```python
from build123d import *
from build123d.topology import SkipClean

# Parameters (mm, degrees)
SKETCH_1_R      = 1.75
EXTRUDE_1_DEPTH = 3
EXTRUDE_START   = 4
SKETCH_2_R      = 9.1
SKETCH_2_R_2    = 7.1
EXTRUDE_2_DEPTH = 4
SKETCH_3_R      = 7.1
SKETCH_3_R_2    = 6.1
EXTRUDE_3_DEPTH = 2


with BuildPart() as part:
    # Эскиз1 → Бобышка-Вытянуть1 (new body)
    # profile 1 of 8: a face of its own
    with BuildSketch(Plane.XY):
        with BuildLine():
            Line((-16, 5), (-16, -5))
            Line((-16, -5), (-7.603288762, -5))
            ThreePointArc((-7.603288762, -5), (-9.1, 0), (-7.603288762, 5))
            Line((-7.603288762, 5), (-16, 5))
        make_face()
        with Locations((-12.5, 0)):
            Circle(SKETCH_1_R, mode=Mode.SUBTRACT)
    # profile 2 of 8: a face of its own
    with BuildSketch(Plane.XY):
        with BuildLine():
            ThreePointArc((-7.603288762, 5), (-9.1, 0), (-7.603288762, -5))
            Line((-7.603288762, -5), (-5.040833264, -5))
            ThreePointArc((-5.040833264, -5), (-7.1, 0), (-5.040833264, 5))
            Line((-5.040833264, 5), (-7.603288762, 5))
        make_face()
    # profile 3 of 8: a face of its own
    with BuildSketch(Plane.XY):
        with BuildLine():
            Line((5.040833264, -5), (7.603288762, -5))
            ThreePointArc((7.603288762, -5), (8.717795815, -2.609604593), (9.1, 0))
            ThreePointArc((9.1, 0), (8.717795815, 2.609604593), (7.603288762, 5))
            Line((7.603288762, 5), (5.040833264, 5))
            ThreePointArc((5.040833264, 5), (6.565055833, 2.703708918), (7.1, 0))
            ThreePointArc((7.1, 0), (6.565055833, -2.703708918), (5.040833264, -5))
        make_face()
    # profile 4 of 8: a face of its own
    with BuildSketch(Plane.XY):
        with BuildLine():
            ThreePointArc((7.603288762, 5), (0, 9.1), (-7.603288762, 5))
            Line((-7.603288762, 5), (-5.040833264, 5))
            ThreePointArc((-5.040833264, 5), (0, 7.1), (5.040833264, 5))
            Line((5.040833264, 5), (7.603288762, 5))
        make_face()
    # profile 5 of 8: a face of its own
    with BuildSketch(Plane.XY):
        with BuildLine():
            ThreePointArc((-7.603288762, 5), (-9.1, 0), (-7.603288762, -5))
            Line((-7.603288762, -5), (-5.040833264, -5))
            ThreePointArc((-5.040833264, -5), (-7.1, 0), (-5.040833264, 5))
            Line((-5.040833264, 5), (-7.603288762, 5))
        make_face()
    # profile 6 of 8: a face of its own
    with BuildSketch(Plane.XY):
        with BuildLine():
            Line((5.040833264, -5), (7.603288762, -5))
            ThreePointArc((7.603288762, -5), (8.717795815, -2.609604593), (9.1, 0))
            ThreePointArc((9.1, 0), (8.717795815, 2.609604593), (7.603288762, 5))
            Line((7.603288762, 5), (5.040833264, 5))
            ThreePointArc((5.040833264, 5), (6.565055833, 2.703708918), (7.1, 0))
            ThreePointArc((7.1, 0), (6.565055833, -2.703708918), (5.040833264, -5))
        make_face()
    # profile 7 of 8: a face of its own
    with BuildSketch(Plane.XY):
        with BuildLine():
            ThreePointArc((9.1, 0), (8.717795815, -2.609604593), (7.603288762, -5))
            Line((7.603288762, -5), (16, -5))
            Line((16, -5), (16, 5))
            Line((16, 5), (7.603288762, 5))
            ThreePointArc((7.603288762, 5), (8.717795815, 2.609604593), (9.1, 0))
        make_face()
        with Locations((12.5, 0)):
            Circle(SKETCH_1_R, mode=Mode.SUBTRACT)
    # profile 8 of 8: a face of its own
    with BuildSketch(Plane.XY):
        with BuildLine():
            Line((-5.040833264, -5), (-7.603288762, -5))
            ThreePointArc((-7.603288762, -5), (0, -9.1), (7.603288762, -5))
            Line((7.603288762, -5), (5.040833264, -5))
            ThreePointArc((5.040833264, -5), (0, -7.1), (-5.040833264, -5))
        make_face()
    extrude(amount=EXTRUDE_1_DEPTH)

    # Эскиз2 → Бобышка-Вытянуть2 (add)
    with SkipClean():  # the faces are left unmerged after this step: merging them gives an invalid solid
        with BuildSketch(Plane(origin=(0, 0, 0), x_dir=(-1, 0, 0), z_dir=(0, 0, -1)).offset(EXTRUDE_START)):
            Circle(SKETCH_2_R)
            Circle(SKETCH_2_R_2, mode=Mode.SUBTRACT)
        extrude(amount=-EXTRUDE_2_DEPTH)

    # Эскиз3 → Бобышка-Вытянуть3 (add)
    with SkipClean():  # the faces are left unmerged after this step: merging them gives an invalid solid
        with BuildSketch(Plane.XY.offset(-4)):
            Circle(SKETCH_3_R)
            Circle(SKETCH_3_R_2, mode=Mode.SUBTRACT)
        extrude(amount=EXTRUDE_3_DEPTH)


solid = part.part
```
Check sheet for the modelled part. Datum: model origin and axes. Units: mm. A direction names the side the tool comes from. Round coordinates to 2 decimals unless told otherwise and drop trailing zeros. Write each loop counter-clockwise with the first axis right and the second up, starting at its lowest first coordinate (ties: lowest second). Pieces come first, ordered by that corner, then holes. Notation, with made-up numbers: (40, -13.75) -> (93, -13.75) arc R23 cw to (93, 12.25) -> close; hole circle Ø4 at (14.5, 2). An arc over 180 degrees is marked (long way). Put each result on its own line as item: value.
(1) Sectioned sample at A-A (x = 12.5). Enter the section's corners in (y, z), plus the area to 3 significant figures.
Values found:
outline: (-5, 0) -> (-1.75, 0) -> (-1.75, 3) -> (-5, 3) -> close; (1.75, 0) -> (5, 0) -> (5, 3) -> (1.75, 3) -> close
area: 19.5 mm^2
(2) Sectioned sample at B-B (y = 3.25). Enter the section's corners in (x, z), plus the area to 3 significant figures.
Values found:
outline: (-16, 0) -> (-8.5, 0) -> (-8.5, -4) -> (-5.16, -4) -> (-5.16, -2) -> (-6.31, -2) -> (-6.31, 3) -> (-16, 3) -> close; (5.16, -4) -> (8.5, -4) -> (8.5, 0) -> (16, 0) -> (16, 3) -> (6.31, 3) -> (6.31, -2) -> (5.16, -2) -> close
area: 80.2 mm^2
(3) Go/stop test with flat-tipped pins: pin 1 Ø4 at (x, y) = (-12.5, 0) entering from -Z; pin 2 Ø0.9 at (x, z) = (-13, 1.5) entering from +Y; pin 3 Ø3 at (x, y) = (12.5, 0) entering from -Z; pin 4 Ø4 at (y, z) = (7, -2) entering from -X. Record where each tip stops, or that it passes through.
Values found:
pin 1: stops at z = 0
pin 2: stops at y = 5
pin 3: passes through
pin 4: stops at x = -7.6
(4) Material ranges on line 1 (Y direction, x = 12.5, z = 1.55); line 2 (X direction, y = 1, z = 1); line 3 (X direction, y = 6, z = 2.5), recorded low to high.
Values found:
line 1: y = -5 to -1.75, 1.75 to 5
line 2: x = -16 to -13.94, -11.06 to -7.03, 7.03 to 11.06, 13.94 to 16
line 3: x = -6.84 to -3.8, 3.8 to 6.84
(5) Tool access check on faces 1 (the face through (-16, 0, 1)), 2 (the face through (12, -5, 1)), 3 (the face through (12, 5, 1)), 4 (the face through (16, 0, 1)), 5 (the face through (2, 6, -2)). Record the directions out of +Z, -Z, +X, -X, +Y, -Y that give a thin tool (end or side, any length) a straight path to the whole face; none if there is none.
Values found:
face 1: +Z, -Z, -X, +Y, -Y
face 2: +Z, -Z, +X, -Y
face 3: +Z, -Z, +X, +Y
face 4: +Z, -Z, +X, +Y, -Y
face 5: +Z
(6) Sectioned sample at D-D (y = 1). Enter the section's corners in (x, z).
Values found:
outline: (-16, 0) -> (-13.94, 0) -> (-13.94, 3) -> (-16, 3) -> close; (-11.06, 0) -> (-9.04, 0) -> (-9.04, -4) -> (-6.02, -4) -> (-6.02, -2) -> (-7.03, -2) -> (-7.03, 3) -> (-11.06, 3) -> close; (6.02, -4) -> (9.04, -4) -> (9.04, 0) -> (11.06, 0) -> (11.06, 3) -> (7.03, 3) -> (7.03, -2) -> (6.02, -2) -> close; (13.94, 0) -> (16, 0) -> (16, 3) -> (13.94, 3) -> close
(7) Sectioned sample at C-C (z = -3). Enter the section's corners in (x, y), plus the area to 3 significant figures.
Values found:
outline: circle Ø18.2 at (0, 0); hole circle Ø12.2 at (0, 0)
area: 143 mm^2
(8) Mould release check, pull along Y, two halves, no side actions. Record for faces 6 (the face through (-10.831, 0.526, 1.479)), 7 (the face through (-12, 5, 1)), 8 (the face through (-12, -5, 1)): released by +Y, released by -Y, zero draft, split by the parting line, or undercut.
Values found:
face 6: undercut
face 7: released by +Y
face 8: released by -Y
